Autodesk Inventor part; units mm, degrees
ref_plane "YZ Plane" through (0, 0, 0) normal (1, 0, 0) x (0, 1, 0)
ref_plane "XZ Plane" through (0, 0, 0) normal (0, 1, 0) x (-1, 0, 0)
ref_plane "XY Plane" through (0, 0, 0) normal (0, 0, 1) x (1, 0, 0)
sketch "Sketch1" plane through (0, 0, 0) normal (0, 0, 1) x (1, 0, 0)
  circle A0 centre (0, 0) radius 1.7526
  dimension "d0" = 3.5052
extrude "Extrusion1" add sketch "Sketch1" along normal blind 6.35
sketch "Sketch2" plane through (0, 0, 0) normal (0, 0, -1) x (-1, 0, 0)
  circle A0 centre (0, 0) radius 1.7526 construction
  circle A1 centre (0, 0) radius 2.8702
  dimension "d3" = 5.7404
extrude "Extrusion2" add sketch "Sketch2" along normal blind 3.5052
sketch "Sketch3" plane through (0, 0, -3.5052) normal (0, 0, -1) x (-1, 0, 0)
  circle A0 centre (0, 0) radius 2.8702
  line L0 (0, 1.604) -> (1.3891, 0.802)
  line L1 (1.3891, 0.802) -> (1.3891, -0.802)
  line L2 (1.3891, -0.802) -> (0, -1.604)
  line L3 (0, -1.604) -> (-1.3891, -0.802)
  line L4 (-1.3891, -0.802) -> (-1.3891, 0.802)
  line L5 (-1.3891, 0.802) -> (0, 1.604)
  dimension "d6" = 2.7781
extrude "Extrusion3" cut sketch "Sketch3" against normal blind 1.7526 contours L0 L1 L2 L3 L4 L5
thread "Thread1"
chamfer "Chamfer1" distance 0.508 angle 45 1 edges at (-1.7526, 0, 6.35)
properties part number "6-32 SHCS x500" material "Stainless Steel"
Geometry check sheet. Reference: the model listing, model coordinates, mm. A direction names the side the tool comes from. Give positions to 0.01 mm unless a question says otherwise; leave off trailing zeros. Write each loop counter-clockwise with the first axis right and the second up, starting at its lowest first coordinate (ties: lowest second). Pieces come first, ordered by that corner, then holes. Notation, with made-up numbers: (-13, 84) - (32, 84) arc R31 cw to (32, 119) - close; hole circle Ø7 at (39, 46.25). An arc over 180 degrees is marked (long way). Put each result on its own line as item: value.
1. Sectioned sample at B-B, the plane z = -1. Enter the section's corners in (x, y), plus the area to 3 significant figures.
Ans:
outline: circle Ø5.74 at (0, 0)
area: 25.9 mm²
2. Go/stop test with flat-tipped pins: pin 1 (1 mm diameter, centred on y = -1.5, z = 3, fed in from -X); pin 2 (3 mm diameter, centred on x = -0.5, z = -0.5, fed in from +Y); pin 3 (1.5 mm diameter, centred on x = -0.5, z = 4.5, fed in from -Y); pin 4 (1.5 mm diameter, centred on y = -2, z = 5.5, fed in from -X). Record where each tip stops, or that it passes through.
Ans:
pin 1: stops at x = -1.44
pin 2: stops at y = 2.87
pin 3: stops at y = -1.75
pin 4: stops at x = -1.23
3. Set-up check for faces 1 (the flat face through (1.389, 0, -3)), 2 (the flat face through (0, 0, 6.35)): record each of +Z, -Z, +X, -X, +Y, -Y from which the full face is reachable in a straight line by a thin tool's end or side.
Ans:
face 1: -Z
face 2: +Z, +X, -X, +Y, -Y
4. Thickness scan on line 1 (Y direction, x = 1.1, z = -3); line 2 (Z direction, x = -0.2, y = 2); line 3 (X direction, y = 0.35, z = -2.75). Record the ranges inside material, lowest first.
Ans:
line 1: y = -2.65 to -0.97, 0.97 to 2.65
line 2: z = -3.51 to 0
line 3: x = -2.85 to -1.39, 1.39 to 2.85
5. Sectioned sample at A-A, the plane y = 0. Enter the section's corners in (x, z), plus the area to 3 significant figures.
Ans:
outline: (-2.87, -3.51) - (-1.39, -3.51) - (-1.39, -1.75) - (1.39, -1.75) - (1.39, -3.51) - (2.87, -3.51) - (2.87, 0) - (1.75, 0) - (1.75, 5.84) - (1.24, 6.35) - (-1.24, 6.35) - (-1.75, 5.84) - (-1.75, 0) - (-2.87, 0) - close
area: 37.3 mm²
6. Sectioned sample at D-D, the plane z = 0.25. Enter the section's corners in (x, y).
Ans:
outline: circle Ø3.51 at (0, 0)
7. Draft check along X on faces 3 (the flat face through (0, 0, -1.753)), 4 (the flat face through (0, -2, 0)), 5 (the cylindrical face through (1.67, -0.53, 2.88)). Enter one of: +X half, -X half, draft (parallel to the pull), parting line (faces both ways), or undercut.
Ans:
face 3: undercut
face 4: draft
face 5: parting line
8. Sectioned sample at C-C, the plane x = -2.05. Enter the section's corners in (y, z).
Ans:
outline: (-2.01, -3.51) - (2.01, -3.51) - (2.01, 0) - (-2.01, 0) - close
